from build123d import *

# Parameters (mm, degrees)
BOSS_EXTRUDE1_DEPTH = 22.86
CHAMFER1_SIZE       = 25.4
CHAMFER1_SIZE_2     = 1.27


with BuildPart() as part:
    # Sketch2 → Boss-Extrude1 (new body)
    with BuildSketch(Plane(origin=(0, 0, 0), x_dir=(1, 0, 0), z_dir=(0, 1, 0))):
        Polygon((-60.96, 5.08), (-59.69, 2.54), (59.69, 2.54), (60.96, 5.08), (60.96, 0), (-60.96, 0), align=None)
    extrude(amount=BOSS_EXTRUDE1_DEPTH)

    # Chamfer1
    # the kernel refuses this chamfer: 25.4, 1.27 mm, written as the material it takes off along each edge
    with BuildSketch(Plane(origin=(-90.492623078, 22.86, -64.145246157), x_dir=(0, -1, 0), z_dir=(0.44721359549995887, 0, 0.8944271909999155))) as chamfer1_piece_1_section:
        Polygon((CHAMFER1_SIZE, 0), (0, -CHAMFER1_SIZE_2), (0, 0), align=None)
    chamfer1_piece_1 = extrude(amount=134.913711846, mode=Mode.PRIVATE)
    chamfer1_piece_1 = split(chamfer1_piece_1, bisect_by=Plane(origin=(-90.492623078, 22.86, -2.54), z_dir=(0, 0, -1)), keep=Keep.TOP, mode=Mode.PRIVATE)
    add(chamfer1_piece_1, mode=Mode.SUBTRACT)
    with BuildSketch(Plane(origin=(-125.726952757, 22.86, -2.54), x_dir=(0, -1, 0), z_dir=(1, 0, 0))) as chamfer1_piece_2_section:
        Polygon((CHAMFER1_SIZE, 0), (0, -CHAMFER1_SIZE_2), (0, 0), align=None)
    chamfer1_piece_2 = extrude(amount=251.453905515, mode=Mode.PRIVATE)
    chamfer1_piece_2 = split(chamfer1_piece_2, bisect_by=Plane(origin=(-72.897390551, 22.86, -28.954781103), z_dir=(0.8944271909999155, 0, -0.44721359549995887)), keep=Keep.TOP, mode=Mode.PRIVATE)
    chamfer1_piece_2 = split(chamfer1_piece_2, bisect_by=Plane(origin=(22.606609449, 22.86, 71.626781103), z_dir=(-0.8944271909999155, 0, -0.44721359549995887)), keep=Keep.TOP, mode=Mode.PRIVATE)
    add(chamfer1_piece_2, mode=Mode.SUBTRACT)
    with BuildSketch(Plane(origin=(30.157376922, 22.86, 56.525246157), x_dir=(0, -1, 0), z_dir=(0.44721359549995887, 0, -0.8944271909999155))) as chamfer1_piece_3_section:
        Polygon((CHAMFER1_SIZE, 0), (0, -CHAMFER1_SIZE_2), (0, 0), align=None)
    chamfer1_piece_3 = extrude(amount=134.913711846, mode=Mode.PRIVATE)
    chamfer1_piece_3 = split(chamfer1_piece_3, bisect_by=Plane(origin=(30.157376922, 22.86, -2.54), z_dir=(0, 0, -1)), keep=Keep.TOP, mode=Mode.PRIVATE)
    add(chamfer1_piece_3, mode=Mode.SUBTRACT)
    with BuildSketch(Plane(origin=(-90.492623078, 22.86, -64.145246157), x_dir=(0, -1, 0), z_dir=(0.44721359549995887, 0, 0.8944271909999155))) as chamfer1_piece_4a_section:
        Polygon((CHAMFER1_SIZE, 0), (0, -CHAMFER1_SIZE_2), (0, 0), align=None)
    chamfer1_piece_4a = extrude(amount=134.913711846, mode=Mode.PRIVATE)
    chamfer1_piece_4a = split(chamfer1_piece_4a, bisect_by=Plane(origin=(-90.492623078, 22.86, -2.54), z_dir=(0, 0, 1)), keep=Keep.TOP, mode=Mode.PRIVATE)
    chamfer1_piece_4a = split(chamfer1_piece_4a, bisect_by=Plane(origin=(-90.492623078, 22.86, 0), z_dir=(0, 0, -1)), keep=Keep.TOP, mode=Mode.PRIVATE)
    chamfer1_piece_4a = split(chamfer1_piece_4a, bisect_by=Plane(origin=(-60.96, 22.86, -64.145246157), z_dir=(1, 0, 0)), keep=Keep.TOP, mode=Mode.PRIVATE)
    chamfer1_piece_4a = split(chamfer1_piece_4a, bisect_by=Plane(origin=(-90.492623078, 0, -64.145246157), z_dir=(0, 1, 0)), keep=Keep.TOP, mode=Mode.PRIVATE)
    with BuildSketch(Plane(origin=(-125.726952757, 22.86, -2.54), x_dir=(0, -1, 0), z_dir=(1, 0, 0))) as chamfer1_piece_4b_section:
        Polygon((CHAMFER1_SIZE, 0), (0, -CHAMFER1_SIZE_2), (0, 0), align=None)
    chamfer1_piece_4b = extrude(amount=251.453905515, mode=Mode.PRIVATE)
    chamfer1_piece_4b = split(chamfer1_piece_4b, bisect_by=Plane(origin=(-72.897390551, 22.86, -28.954781103), z_dir=(-0.8944271909999155, 0, 0.44721359549995887)), keep=Keep.TOP, mode=Mode.PRIVATE)
    chamfer1_piece_4b = split(chamfer1_piece_4b, bisect_by=Plane(origin=(-60.96, 22.86, -2.54), z_dir=(1, 0, 0)), keep=Keep.TOP, mode=Mode.PRIVATE)
    chamfer1_piece_4b = split(chamfer1_piece_4b, bisect_by=Plane(origin=(-125.726952757, 0, -2.54), z_dir=(0, 1, 0)), keep=Keep.TOP, mode=Mode.PRIVATE)
    chamfer1_piece_4 = chamfer1_piece_4a & chamfer1_piece_4b
    add(chamfer1_piece_4, mode=Mode.SUBTRACT)
    with BuildSketch(Plane(origin=(-125.726952757, 22.86, -2.54), x_dir=(0, -1, 0), z_dir=(1, 0, 0))) as chamfer1_piece_5a_section:
        Polygon((CHAMFER1_SIZE, 0), (0, -CHAMFER1_SIZE_2), (0, 0), align=None)
    chamfer1_piece_5a = extrude(amount=251.453905515, mode=Mode.PRIVATE)
    chamfer1_piece_5a = split(chamfer1_piece_5a, bisect_by=Plane(origin=(22.606609449, 22.86, 71.626781103), z_dir=(0.8944271909999155, 0, 0.44721359549995887)), keep=Keep.TOP, mode=Mode.PRIVATE)
    chamfer1_piece_5a = split(chamfer1_piece_5a, bisect_by=Plane(origin=(60.96, 22.86, -2.54), z_dir=(-1, 0, 0)), keep=Keep.TOP, mode=Mode.PRIVATE)
    chamfer1_piece_5a = split(chamfer1_piece_5a, bisect_by=Plane(origin=(-125.726952757, 0, -2.54), z_dir=(0, 1, 0)), keep=Keep.TOP, mode=Mode.PRIVATE)
    with BuildSketch(Plane(origin=(30.157376922, 22.86, 56.525246157), x_dir=(0, -1, 0), z_dir=(0.44721359549995887, 0, -0.8944271909999155))) as chamfer1_piece_5b_section:
        Polygon((CHAMFER1_SIZE, 0), (0, -CHAMFER1_SIZE_2), (0, 0), align=None)
    chamfer1_piece_5b = extrude(amount=134.913711846, mode=Mode.PRIVATE)
    chamfer1_piece_5b = split(chamfer1_piece_5b, bisect_by=Plane(origin=(30.157376922, 22.86, -2.54), z_dir=(0, 0, 1)), keep=Keep.TOP, mode=Mode.PRIVATE)
    chamfer1_piece_5b = split(chamfer1_piece_5b, bisect_by=Plane(origin=(60.96, 22.86, 56.525246157), z_dir=(-1, 0, 0)), keep=Keep.TOP, mode=Mode.PRIVATE)
    chamfer1_piece_5b = split(chamfer1_piece_5b, bisect_by=Plane(origin=(30.157376922, 22.86, 0), z_dir=(0, 0, -1)), keep=Keep.TOP, mode=Mode.PRIVATE)
    chamfer1_piece_5b = split(chamfer1_piece_5b, bisect_by=Plane(origin=(30.157376922, 0, 56.525246157), z_dir=(0, 1, 0)), keep=Keep.TOP, mode=Mode.PRIVATE)
    chamfer1_piece_5 = chamfer1_piece_5a & chamfer1_piece_5b
    add(chamfer1_piece_5, mode=Mode.SUBTRACT)


solid = part.part
Input: part model. Units: mm. Frame: model coordinates. A direction names the side the tool comes from. Coordinates: 2 decimals unless noted, no trailing zeros. Loops run counter-clockwise (first coordinate to the right, second up) from the corner with the lowest first, then second, coordinate; pieces in that order, holes last.
(1) First-contact query: pin 1 Ø1.5 at (x, y) = (-45, 11) entering from -Z; pin 2 Ø10 at (x, y) = (-12, 14) entering from +Z; pin 3 Ø1.5 at (x, y) = (-6, 3) entering from -Z; pin 4 Ø1.5 at (x, z) = (8.5, -3.5) entering from +Y. Flat tips, straight axial feed; report the tip coordinate or a pass-through.
(2) Section D-D on y = 5.75. Return the cut outline in (x, z).
(3) Section C-C on x = -10.5. Return the cut outline in (y, z).
(4) Set-up query: faces 1 (the face through (60.96, 9, -2)), 2 (the face through (-0.85, 11.27, -1.85)). Return all of +Z, -Z, +X, -X, +Y, -Y with unobstructed straight access to the full face (end or side cutting, diameter ignored); none if empty.
(5) Material intervals for probe 1 along Z at (x, y) = (53, 3.75); probe 2 along X at (y, z) = (4.25, -2.7); probe 3 along Z at (x, y) = (-3, 3), sorted ascending.
(6) Section A-A on z = -3.6. Return the cut outline in (x, y).
(7) Section B-B on y = 16.25. Return the cut outline in (x, z).
Data:
1. pin 1: stops at z = -1.9
1. pin 2: stops at z = 0
1. pin 3: stops at z = -2.3
1. pin 4: passes through
2. outline: (-60.96, -4.15) - (-59.95, -2.13) - (59.95, -2.13) - (60.96, -4.15) - (60.96, 0) - (-60.96, 0) - close
3. outline: (0, -2.41) - (22.86, -1.27) - (22.86, 0) - (0, 0) - close
4. face 1: +Z, -Z, +X, +Y, -Y
4. face 2: -Z, +Y
5. probe 1: z = -2.23 to 0
5. probe 2: x = -60.96 to -60.15, 60.15 to 60.96
5. probe 3: z = -2.26 to 0
6. outline: (-60.96, 0) - (-60.36, 0) - (-60.96, 10.7) - close; (60.36, 0) - (60.96, 0) - (60.96, 10.7) - close
7. outline: (-60.96, -2.98) - (-60.27, -1.6) - (60.27, -1.6) - (60.96, -2.98) - (60.96, 0) - (-60.96, 0) - close
